Design review of the part shown in the three views and the two pictorial views. Dimensions are in mm from the part's minimum x, y and z. Round coordinates to 2 decimals unless told otherwise and drop trailing zeros. Order: outer loops, then holes, each group sorted by start corner. A loop starts at its lowest first (then second) coordinate and runs counter-clockwise, first axis right, second up. Notation, with made-up numbers: (19.25, -1) - (27.25, -1) arc R24 ccw to (27.25, 37) - close; hole circle Ø6 at (47, 81.25). An arc over 180 degrees is marked (long way). Use CSV: the item, a comma, the result in double quotes.
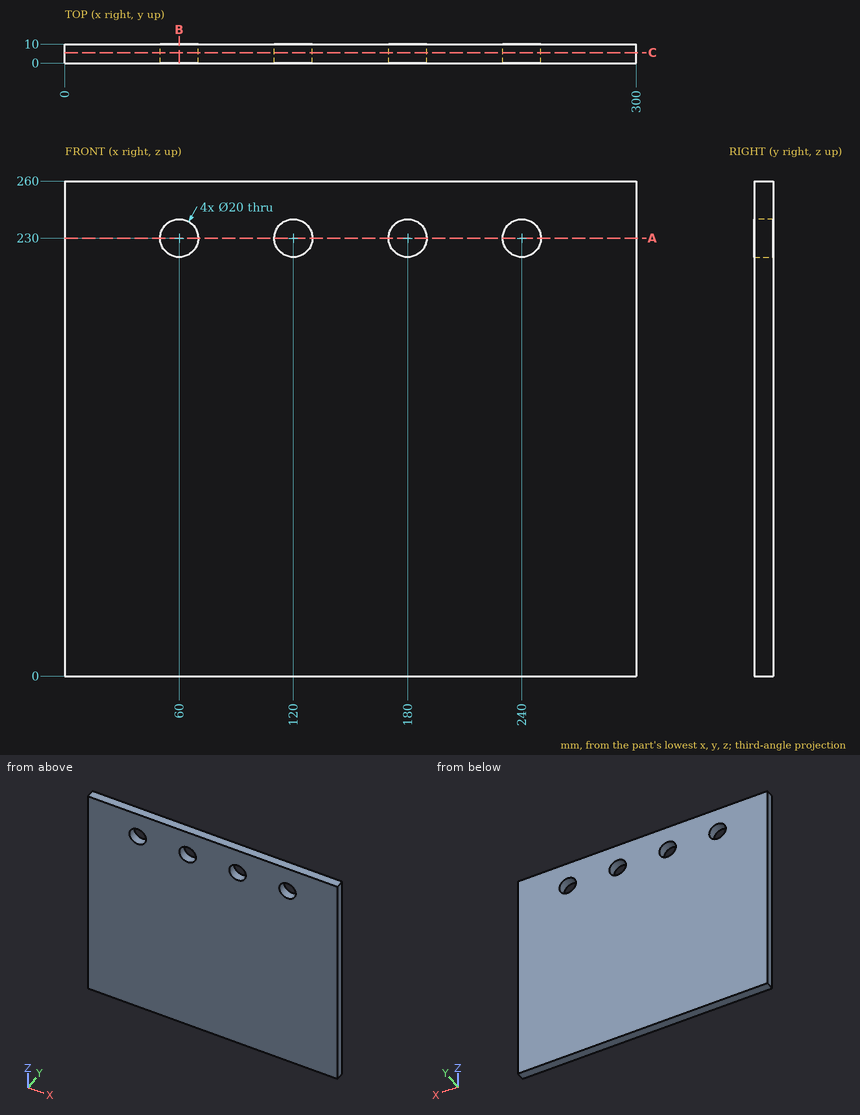
1) To check wall thickness, follow L1, parallel to X at y = 4.75, z = 230; L2, parallel to Z at x = 179, y = 6.5; L3, parallel to Z at x = 111, y = 5.75. State the ranges of each line that lie inside material, in increasing order. Write a range as from..to.
Data:
L1,"x = 0..50, 70..110, 130..170, 190..230, 250..300"
L2,"z = 0..220.05, 239.95..260"
L3,"z = 0..225.64, 234.36..260"
2) We need section A-A (z = 230). Give the boundary of the cut face in (x, y), then the cut area to 3 significant figures.
Data:
outline,"(0, 0) - (50, 0) - (50, 10) - (0, 10) - close; (70, 0) - (110, 0) - (110, 10) - (70, 10) - close; (130, 0) - (170, 0) - (170, 10) - (130, 10) - close; (190, 0) - (230, 0) - (230, 10) - (190, 10) - close; (250, 0) - (300, 0) - (300, 10) - (250, 10) - close"
area,"2,200 mm2"
3) We need section C-C (y = 5.5). Give the boundary of the cut face in (x, z), then the cut area to 3 significant figures.
Data:
outline,"(0, 0) - (300, 0) - (300, 260) - (0, 260) - close; hole circle Ø20 at (60, 230); hole circle Ø20 at (120, 230); hole circle Ø20 at (180, 230); hole circle Ø20 at (240, 230)"
area,"76,700 mm2"
4) We need section B-B (x = 60). Give the boundary of the cut face in (y, z).
Data:
outline,"(0, 0) - (10, 0) - (10, 220) - (0, 220) - close; (0, 240) - (10, 240) - (10, 260) - (0, 260) - close"
